```python
from build123d import *

# Parameters (mm, degrees)
SKETCH1_R           = 1.5
SKETCH1_W           = 30.7
SKETCH1_H           = 30.7
BOSS_EXTRUDE1_DEPTH = 2
BOSS_EXTRUDE2_DEPTH = 4


with BuildPart() as part:
    # Sketch1 → Boss-Extrude1 (new body)
    with BuildSketch(Plane(origin=(0, 0, 0), x_dir=(1, 0, 0), z_dir=(0, 1, 0))):
        Polygon((-22.005550203, -21.814567772), (-14.005550203, -21.814567772), (16.694449797, -21.814567772), (24.694449797, -21.814567772), (24.694449797, -13.814567772), (24.694449797, 16.669052986), (24.694449797, 24.885432228), (-22.005550203, 24.885432228), (-22.005550203, 15.385432228), (-22.005550203, -15.314567772), align=None)
        with Locations(Location((-16.905550203, 19.785432228, 0), (0, 0, 270))):
            Circle(SKETCH1_R, mode=Mode.SUBTRACT)
        with Locations(Location((-16.905550203, -16.714567772, 0), (0, 0, 270))):
            Circle(SKETCH1_R, mode=Mode.SUBTRACT)
        with Locations(Location((19.594449797, 19.785432228, 0), (0, 0, 270))):
            Circle(SKETCH1_R, mode=Mode.SUBTRACT)
        with Locations(Location((19.594449797, -16.714567772, 0), (0, 0, 270))):
            Circle(SKETCH1_R, mode=Mode.SUBTRACT)
        with Locations((1.344449797, 1.535432228)):
            Rectangle(SKETCH1_W, SKETCH1_H, mode=Mode.SUBTRACT)
    extrude(amount=BOSS_EXTRUDE1_DEPTH)

    # Sketch3 → Boss-Extrude2 (add)
    with BuildSketch(Plane(origin=(0, 0, 0), x_dir=(1, 0, 0), z_dir=(0, 1, 0))):
        Polygon((-14.205550203, 24.885432228), (-14.205550203, 26.885432228), (-24.205550203, 26.885432228), (-24.205550203, 16.885432228), (-22.205550203, 16.885432228), (-22.205550203, 24.885432228), align=None)
        Polygon((-22.005550203, -13.814567772), (-24.205550203, -13.814567772), (-24.205550203, -23.814567772), (-14.005550203, -23.814567772), (-14.005550203, -21.814567772), (-22.005550203, -21.814567772), align=None)
        Polygon((15.994449797, 26.885432228), (26.494449797, 26.885432228), (26.494449797, 16.885432228), (24.494449797, 16.885432228), (24.494449797, 24.885432228), (15.994449797, 24.885432228), align=None)
        Polygon((16.694449797, -21.814567772), (16.694449797, -23.814567772), (26.494449797, -23.814567772), (26.494449797, -13.814567772), (24.694449797, -13.814567772), (24.694449797, -21.814567772), align=None)
    extrude(amount=BOSS_EXTRUDE2_DEPTH)


solid = part.part
```
Verification items for the finished model (mm, model axes). A direction names the side the tool comes from. Round coordinates to 2 decimals unless told otherwise and drop trailing zeros. Loops run counter-clockwise (first coordinate to the right, second up) from the corner with the lowest first, then second, coordinate; pieces in that order, holes last. Notation, with made-up numbers: (-2, -37.75) -> (32, -37.75) arc R16 cw to (32, -26.75) -> close; hole circle Ø1 at (55.25, -12). An arc over 180 degrees is marked (long way). Answer as a JSON object with one key per item and string values.
Q1. Draft check along Z on faces 1 (the flat face through (21, 3, 21.815)), 2 (the flat face through (-24.206, 2, -22)), 3 (the flat face through (1, 1, 21.815)). Enter one of: pulls with the +Z half, pulls with the -Z half, needs draft (parallel to the pull), parting line crosses it, or undercut.
Data:
{"face 1": "undercut", "face 2": "needs draft", "face 3": "pulls with the +Z half"}
Q2. Access from +Z, -Z, +X, -X, +Y, -Y to the whole of each face (thin tool, end or side, straight path). Record for faces 4 (the flat face through (20, 3, -24.885)), 5 (the flat face through (-22.006, 1, -6)), 6 (the flat face through (-14.006, 2, 23)), 7 (the flat face through (26, 2, 13.815)).
Data:
{"face 4": "+Y", "face 5": "+Y, -Y", "face 6": "+Z, +Y, -Y", "face 7": "+X, +Y, -Y"}
Q3. Section check C-C (z = -9). Record the boundary of the cut face in (x, y).
Data:
{"outline": "(-22.01, 0) -> (-14.01, 0) -> (-14.01, 2) -> (-22.01, 2) -> close; (16.69, 0) -> (24.69, 0) -> (24.69, 2) -> (16.69, 2) -> close"}
Q4. Section check A-A (x = -1). Record the boundary of the cut face in (y, z), then the cut area to 3 significant figures.
Data:
{"outline": "(0, -24.89) -> (2, -24.89) -> (2, -16.89) -> (0, -16.89) -> close; (0, 13.81) -> (2, 13.81) -> (2, 21.81) -> (0, 21.81) -> close", "area": "32.0 mm2"}
Q5. Section check B-B (y = 3.4). Record the boundary of the cut face in (x, z), then the cut area to 3 significant figures.
Data:
{"outline": "(-24.21, -26.89) -> (-14.21, -26.89) -> (-14.21, -24.89) -> (-22.21, -24.89) -> (-22.21, -16.89) -> (-24.21, -16.89) -> close; (-24.21, 13.81) -> (-22.01, 13.81) -> (-22.01, 21.81) -> (-14.01, 21.81) -> (-14.01, 23.81) -> (-24.21, 23.81) -> close; (15.99, -26.89) -> (26.49, -26.89) -> (26.49, -16.89) -> (24.49, -16.89) -> (24.49, -24.89) -> (15.99, -24.89) -> close; (16.69, 21.81) -> (24.69, 21.81) -> (24.69, 13.81) -> (26.49, 13.81) -> (26.49, 23.81) -> (16.69, 23.81) -> close", "area": "145 mm2"}
Q6. Scan lines: line 1 (X direction, y = 1.5, z = 7); line 2 (Z direction, x = -6, y = 1.95); line 3 (Z direction, x = -20.5, y = 2.55). Record each from-to range of solid material in increasing order. Write a range as from..to.
Data:
{"line 1": "x = -22.01..-14.01, 16.69..24.69", "line 2": "z = -24.89..-16.89, 13.81..21.81", "line 3": "z = -26.89..-24.89, 21.81..23.81"}
Q7. Go/stop test with flat-tipped pins: P1, Ø2, axis at y = 1.5, z = -8.5, coming from the -X side; P2, Ø1, axis at x = 10.5, y = 3.5, coming from the +Z side; P3, Ø1, axis at y = 1.5, z = -9, coming from the +X side; P4, Ø4, axis at x = -10.5, z = -17, coming from the +Y side. Record where each tip stops, or that it passes through.
Data:
{"P1": "stops at x = -22.01", "P2": "passes through", "P3": "stops at x = 24.69", "P4": "stops at y = 2"}
Q8. Section check D-D (x = 23). Record the boundary of the cut face in (y, z).
Data:
{"outline": "(0, -26.89) -> (4, -26.89) -> (4, -24.89) -> (2, -24.89) -> (2, 21.81) -> (4, 21.81) -> (4, 23.81) -> (0, 23.81) -> close"}
